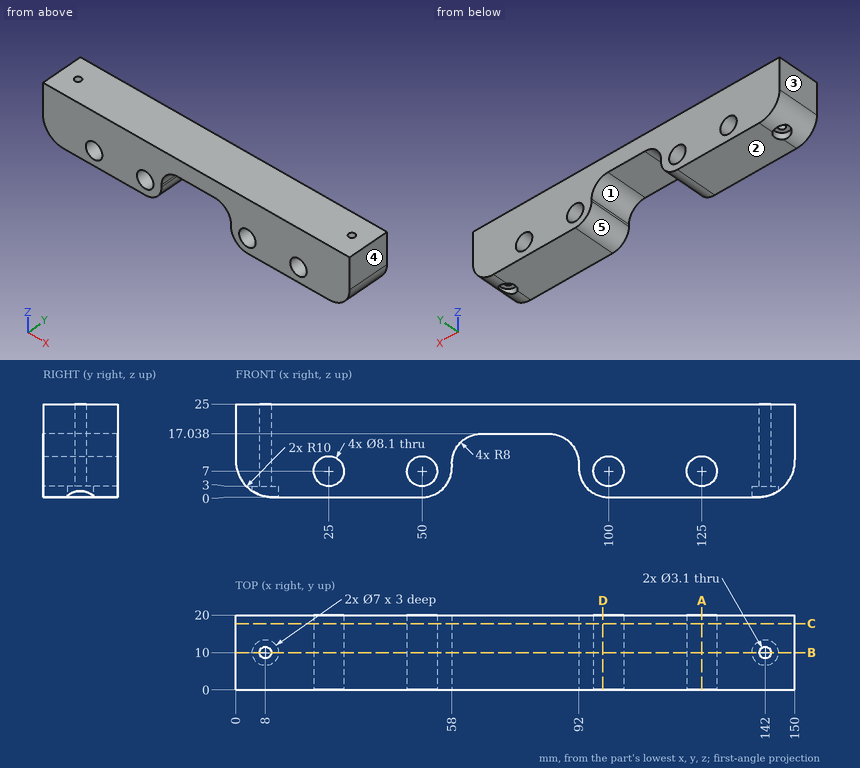
Study the drawing (mm; zero at the part's minimum x, y, z) and answer. A direction names the side the tool comes from. Give positions to 0.01 mm unless a question says otherwise; leave off trailing zeros. Write each loop counter-clockwise with the first axis right and the second up, starting at its lowest first coordinate (ties: lowest second). Pieces come first, ordered by that corner, then holes. Notation, with made-up numbers: (68, -25) - (105, -25) arc R24 cw to (105, 10) - close; hole circle Ø11 at (14.5, 26.25). An arc over 180 degrees is marked (long way). Use a Markdown table: item, result.
1. Section B-B on y = 10 is taken. Count the separate pieces of the cut face and the enclosed holes in it, plus the area to 3 significant figures.
Values follow:
| item | result |
|---|---|
| separate pieces | 3 |
| enclosed holes | 4 |
| area | 2,750 mm² |
2. For a pull along X with two mould halves and no side action, classify the marked faces 3, 4 and 5 as released by +X, released by -X, zero draft, split by the parting line, or undercut.
Values follow:
| item | result |
|---|---|
| face 3 | released by -X |
| face 4 | released by +X |
| face 5 | undercut |
3. Section D-D on x = 98.5 is taken. Write down the section's boundary in (y, z), plus the area to 3 significant figures.
Values follow:
| item | result |
|---|---|
| outline | (0, 0.14) - (20, 0.14) - (20, 3.24) - (0, 3.24) - close; (0, 10.76) - (20, 10.76) - (20, 25) - (0, 25) - close |
| area | 347 mm² |
4. Section C-C on y = 17.75 is taken. Write down the section's boundary in (x, z).
Values follow:
| item | result |
|---|---|
| outline | (0, 10) arc R10 ccw to (10, 0) - (50, 0) arc R8 ccw to (58, 8) - (58, 9.04) arc R8 cw to (66, 17.04) - (84, 17.04) arc R8 cw to (92, 9.04) - (92, 8) arc R8 ccw to (100, 0) - (140, 0) arc R10 ccw to (150, 10) - (150, 25) - (0, 25) - close; hole circle Ø8.1 at (25, 7); hole circle Ø8.1 at (50, 7); hole circle Ø8.1 at (100, 7); hole circle Ø8.1 at (125, 7) |
5. Each of these flat-tipped pins is pushed along its axis until it touches: P1, Ø1.5, axis at x = 76, z = 16.5, coming from the -Y side; P2, Ø5.5, axis at x = 7.5, y = 9, coming from the -Z side; P3, Ø5.5, axis at x = 8, y = 10, coming from the -Z side; P4, Ø0.5, axis at y = 12, z = 8.5, coming from the -X side. Where does it stop, or does it pass through?
Values follow:
| item | result |
|---|---|
| P1 | stops at y = 0 |
| P2 | stops at z = 0.07 |
| P3 | stops at z = 3 |
| P4 | stops at x = 0.08 |
6. Section A-A on x = 125 is taken. Write down the section's boundary in (y, z), plus the area to 3 significant figures.
Values follow:
| item | result |
|---|---|
| outline | (0, 0) - (20, 0) - (20, 2.95) - (0, 2.95) - close; (0, 11.05) - (20, 11.05) - (20, 25) - (0, 25) - close |
| area | 338 mm² |
7. Find the intervals of material crossed by probe 1 along X at (y, z) = (17.25, 9.25); probe 2 along Y at (x, z) = (142, 1.75); probe 3 along Y at (x, z) = (8, 9.5), in increasing order. Write a range as from..to.
Values follow:
| item | result |
|---|---|
| probe 1 | x = 0.03..21.63, 28.37..46.63, 53.37..58, 92..96.63, 103.37..121.63, 128.37..149.97 |
| probe 2 | y = 0..6.5, 13.5..20 |
| probe 3 | y = 0..8.45, 11.55..20 |
8. A tool of negligible diameter and unlimited length cuts with its end or side. For the marked faces 1 and 2, from which of +Z, -Z, +X, -X, +Y, -Y can it reach the whole face along a straight path? Write none if from no direction.
Values follow:
| item | result |
|---|---|
| face 1 | -Z, +Y, -Y |
| face 2 | -Z, +X, -X, +Y, -Y |
